Here's the drawing with two shaded views (mm, measured from the low corner). I have some questions. A direction names the side the tool comes from. Coordinates: 2 decimals unless noted, no trailing zeros. Write each loop counter-clockwise with the first axis right and the second up, starting at its lowest first coordinate (ties: lowest second). Pieces come first, ordered by that corner, then holes. Notation, with made-up numbers: (-6.75, 33) - (16.25, 33) arc R12 ccw to (16.25, 46) - close; hole circle Ø9 at (-12.75, 89). An arc over 180 degrees is marked (long way). Answer in a Markdown table with one row per item. Add a question column.
Item 1: Imagine slicing it at C-C (x = 14). Please give me the cut outline in (y, z).
Item 2: I'm going to push flat-ended pins straight in: pin 1 (2.5 mm diameter, centred on x = 7.5, z = 4.5, fed in from -Y); pin 2 (4 mm diameter, centred on y = 5.5, z = 2.5, fed in from -X); pin 3 (2 mm diameter, centred on x = 15.5, y = 1.5, fed in from +Z); pin 4 (0.5 mm diameter, centred on x = 11.5, z = 7.5, fed in from -Y). Where does each tip first touch, or does it pass through?
Item 3: If I drill on probe 1 along X at (y, z) = (0.5, 7); probe 2 along Z at (x, y) = (2.5, 4.5); probe 3 along Y at (x, z) = (11.5, 5), over which ranges is the centre line in solid material (lowest first)? Write a range as from..to.
Item 4: Imagine slicing it at B-B (z = 6.75). Please give me the cut outline in (x, y).
Item 5: We'd pull the mould along X, two halves only. Please class the marked faces 3, 4, 5 and 6: +X half, -X half, draft (parallel to the pull), parting line (faces both ways), or undercut.
Item 6: Which directions (+Z, -Z, +X, -X, +Y, -Y) give clear straight access to the entire face, cutting with the end or side of a thin tool? Please do the marked faces 1 and 2.
Item 7: Imagine slicing it at D-D (y = 2). Please give me the cut outline in (x, z).
Item 8: Imagine slicing it at A-A (y = 5.5). Please give me the cut outline in (x, z).
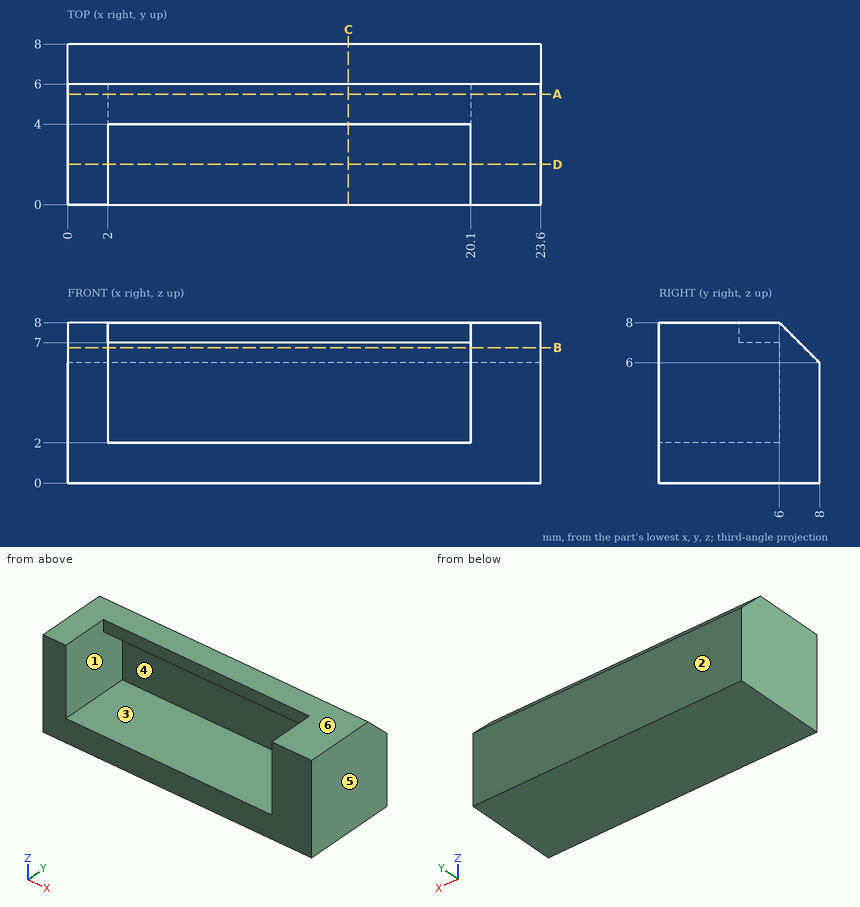
Here are the results:
| question | item | result |
|---|---|---|
| 1 | outline | (0, 0) - (8, 0) - (8, 6) - (6, 8) - (4, 8) - (4, 7) - (6, 7) - (6, 2) - (0, 2) - close |
| 2 | pin 1 | stops at y = 6 |
| 2 | pin 2 | stops at x = 0 |
| 2 | pin 3 | stops at z = 2 |
| 2 | pin 4 | stops at y = 4 |
| 3 | probe 1 | x = 0..2, 20.1..23.6 |
| 3 | probe 2 | z = 0..2, 7..8 |
| 3 | probe 3 | y = 6..8 |
| 4 | outline | (0, 0) - (2, 0) - (2, 6) - (20.1, 6) - (20.1, 0) - (23.6, 0) - (23.6, 7.25) - (0, 7.25) - close |
| 5 | face 3 | undercut |
| 5 | face 4 | undercut |
| 5 | face 5 | +X half |
| 5 | face 6 | draft |
| 6 | face 1 | -Y |
| 6 | face 2 | +Z, -Z, +X, -X, +Y |
| 7 | outline | (0, 0) - (23.6, 0) - (23.6, 8) - (20.1, 8) - (20.1, 2) - (2, 2) - (2, 8) - (0, 8) - close |
| 8 | outline | (0, 0) - (23.6, 0) - (23.6, 8) - (0, 8) - close; hole (2, 2) - (20.1, 2) - (20.1, 7) - (2, 7) - close |
